Check sheet for the modelled part. Datum: model origin and axes. Units: mm. A direction names the side the tool comes from. Give positions to 0.01 mm unless a question says otherwise; leave off trailing zeros. Write each loop counter-clockwise with the first axis right and the second up, starting at its lowest first coordinate (ties: lowest second). Pieces come first, ordered by that corner, then holes.
Autodesk Inventor part; units mm, degrees
sketch "Sketch2" plane through (0, 0, 0) normal (1, 0, 0) x (0, 1, 0)
  line L0 (13.85, 0.8) -> (-13.85, 0.8)
  line L1 (-13.85, 0.8) -> (-13.85, -0.8)
  line L2 (-13.85, -0.8) -> (18.65, -0.8)
  line L3 (18.65, -0.8) -> (18.65, 0.8)
  line L4 (0, 4.96) -> (0, -1.76)
  line L5 (-20.95, 0) -> (28.75, 0)
  line L6 (18.65, 0.8) -> (21.65, 0.8)
  line L7 (21.65, 0.8) -> (21.65, 4)
  line L8 (21.65, 4) -> (20.05, 4)
  line L9 (20.05, 4) -> (20.05, 2.4)
  line L10 (20.05, 2.4) -> (18.65, 2.4)
  line L11 (18.65, 2.4) -> (18.65, 4)
  line L12 (18.65, 4) -> (17.05, 4)
  line L13 (17.05, 4) -> (17.05, 4)
  arc A0 (13.85, 0.8) -> (17.05, 4) centre (13.85, 4) ccw
  point P0 (0, 0)
  point P1 (0, 0.8)
  point P2 (18.65, 0)
  dimension "d0" = 32.5
  dimension "d1" = 1.6
  dimension "d2" = 3
  dimension "d3" = 3.2
  dimension "d4" = 1.6
  dimension "d6" = 1.6
  dimension "d7" = 1.6
  dimension "d8" = 1.4
  dimension "d12" = 1.6
  dimension "d13" = 3.2
extrude "Extrusion1" add sketch "Sketch2" along normal mid plane 100
equation "\"d13\" = d3"
properties part number "Hanging_Wall"
1) Gauge pin test, flat ends, axial feed: pin 1 (14 mm diameter, centred on x = -13.5, y = -5, fed in from +Z); pin 2 (3.5 mm diameter, centred on x = 22.5, y = 19.5, fed in from -Z); pin 3 (1.8 mm diameter, centred on x = 20, z = 3, fed in from -Y); pin 4 (1.8 mm diameter, centred on x = 18.5, z = -0.5, fed in from +Y). Record the tip position at first contact, or that the pin passes through.
2) Draft check along Y on faces 1 (the flat face through (-1, 18.65, 0)), 2 (the flat face through (-1, 18, 4)), 3 (the flat face through (-1, 20.05, 3)). Enter one of: +Y half, -Y half, draft (parallel to the pull), parting line (faces both ways), or undercut.
3) Sectioned sample at A-A on x = -10. Record the boundary of the cut face in (y, z).
4) Access from +Z, -Z, +X, -X, +Y, -Y to the whole of each face (thin tool, end or side, straight path). Record for faces 4 (the flat face through (-1, 0, 0.8)), 5 (the flat face through (-1, 18.65, 3)), 6 (the flat face through (-1, 20, 0.8)).
5) Scan lines: L1, parallel to Z at x = 9, y = 0; L2, parallel to Y at x = 15, z = 3.05; L3, parallel to Y at x = -18, z = 0.3. Record each from-to range of solid material in increasing order.
6) Sectioned sample at B-B on z = 3.15. Record the boundary of the cut face in (x, y), then the cut area to 3 significant figures.
7) Sectioned sample at C-C on y = 9.5. Record the boundary of the cut face in (x, z), then the cut area to 3 significant figures.
Answers below:
1. pin 1: stops at z = 0.8
1. pin 2: stops at z = -0.8
1. pin 3: stops at y = 16.42
1. pin 4: stops at y = 18.65
2. face 1: +Y half
2. face 2: draft
2. face 3: undercut
3. outline: (-13.85, -0.8) - (18.65, -0.8) - (18.65, 0.8) - (21.65, 0.8) - (21.65, 4) - (20.05, 4) - (20.05, 2.4) - (18.65, 2.4) - (18.65, 4) - (17.05, 4) arc R3.2 cw to (13.85, 0.8) - (-13.85, 0.8) - close
4. face 4: +Z, +X, -X, -Y
4. face 5: +Z, +X, -X
4. face 6: -Z, +X, -X, +Y
5. L1: z = -0.8 to 0.8
5. L2: y = 16.91 to 18.65, 20.05 to 21.65
5. L3: y = -13.85 to 18.65
6. outline: (-50, 16.94) - (50, 16.94) - (50, 18.65) - (-50, 18.65) - close; (-50, 20.05) - (50, 20.05) - (50, 21.65) - (-50, 21.65) - close
6. area: 331 mm2
7. outline: (-50, -0.8) - (50, -0.8) - (50, 0.8) - (-50, 0.8) - close
7. area: 160 mm2
